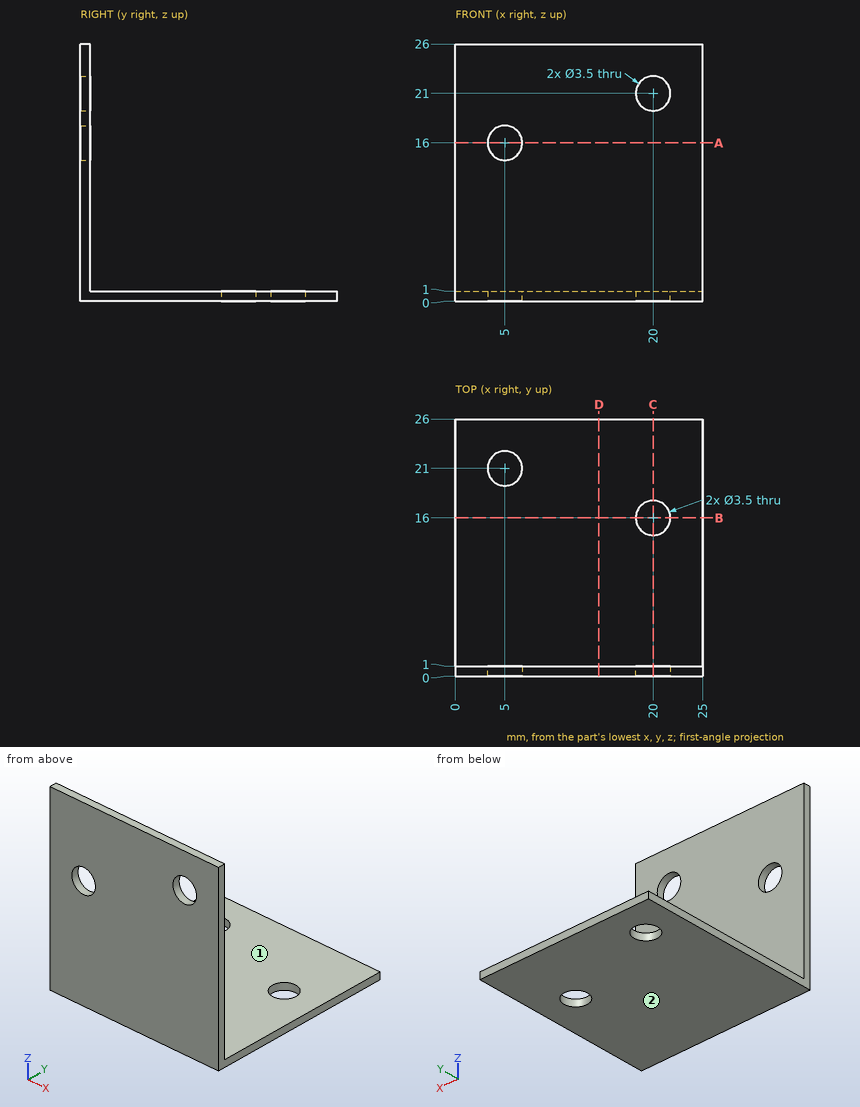
The figure shows three views and two pictorial views of one solid part (mm, origin at its lowest corner). Answer the questions. A direction names the side the tool comes from. Coordinates: 2 decimals unless noted, no trailing zeros. Order: outer loops, then holes, each group sorted by start corner. A loop starts at its lowest first (then second) coordinate and runs counter-clockwise, first axis right, second up.
Q1. Given P1, Ø3, axis at x = 17, y = 9.5, coming from the +Z side; P2, Ø4, axis at x = 20, z = 21, coming from the +Y side, each flat-ended and moving along its own axis, determine where each tip first touches the part or whether it passes through.
Q2. A cutting plane is placed at A-A, the plane z = 16. Write down the section's boundary in (x, y).
Q3. Which of the six approach directions +Z, -Z, +X, -X, +Y, -Y give full straight-line access (tool end or side, diameter ignored) to the marked faces 1 and 2?
Q4. A cutting plane is placed at B-B, the plane y = 16. Write down the section's boundary in (x, z).
Q5. A cutting plane is placed at C-C, the plane x = 20. Write down the section's boundary in (y, z).
Q6. Consider line 1 (Z direction, x = 5, y = 0.45); line 2 (Z direction, x = 20, y = 0.7). Determine where each line is inside the solid, lowest interval first.
Q7. A cutting plane is placed at D-D, the plane x = 14.5. Write down the section's boundary in (y, z), and give its area (3 significant figures).
Answers follow:
1. P1: stops at z = 1
1. P2: stops at y = 1
2. outline: (0, 0) - (3.25, 0) - (3.25, 1) - (0, 1) - close; (6.75, 0) - (25, 0) - (25, 1) - (6.75, 1) - close
3. face 1: +Z, +X, -X, +Y
3. face 2: -Z, +X, -X, +Y, -Y
4. outline: (0, 0) - (18.25, 0) - (18.25, 1) - (0, 1) - close; (21.75, 0) - (25, 0) - (25, 1) - (21.75, 1) - close
5. outline: (0, 0) - (14.25, 0) - (14.25, 1) - (1, 1) - (1, 19.25) - (0, 19.25) - close; (0, 22.75) - (1, 22.75) - (1, 26) - (0, 26) - close; (17.75, 0) - (26, 0) - (26, 1) - (17.75, 1) - close
6. line 1: z = 0 to 14.25, 17.75 to 26
6. line 2: z = 0 to 19.25, 22.75 to 26
7. outline: (0, 0) - (26, 0) - (26, 1) - (1, 1) - (1, 26) - (0, 26) - close
7. area: 51.0 mm2
